Autodesk Inventor part; units mm, degrees
ref_plane "BODY_N_XY" through (62, 0, 0) normal (0, 0, -1) x (1, 0, 0)
ref_plane "BODY_N_YZ" through (62, 0, 0) normal (1, 0, 0) x (0, -1, 0)
ref_plane "BODY_N_ZX" through (62, 0, 0) normal (0, -1, 0) x (0, 0, -1)
sketch "Sketch_8" plane through (0, 0, 0) normal (0, 0, 1) x (1, 0, 0)
  line L0 (0, 0) -> (-8, 0)
  line L1 (-8, 0) -> (-8, 4.3865)
  line L2 (-8, 4.3865) -> (-7.3865, 5)
  line L3 (-7.3865, 5) -> (0, 5)
  line L4 (0, 5) -> (0, 0)
  line L5 (0, 0) -> (-8, 0)
revolve "Revolution1" add sketch "Sketch_8" angle 360 about axis through (0, 0, 0) along (1, 0, 0)
thread "Thread1"
sketch "Sketch_9" plane through (0, 0, 0) normal (1, 0, 0) x (0, 0, -1)
  line L0 (-9.15, 4.0345) -> (-9.15, -4.0345)
  arc A0 (-9.15, -4.0345) -> (-4.0345, -9.15) centre (0, 0) ccw
  line L1 (-4.0345, -9.15) -> (4.0345, -9.15)
  arc A1 (4.0345, -9.15) -> (9.15, -4.0345) centre (0, 0) ccw
  line L2 (9.15, -4.0345) -> (9.15, 4.0345)
  arc A2 (9.15, 4.0345) -> (4.0345, 9.15) centre (0, 0) ccw
  line L3 (4.0345, 9.15) -> (-4.0345, 9.15)
  arc A3 (-4.0345, 9.15) -> (-9.15, 4.0345) centre (0, 0) ccw
extrude "Extrusion1" add sketch "Sketch_9" along normal blind 12.5
sketch "Sketch_11" plane through (12.5, 0, 0) normal (1, 0, 0) x (0, 0, -1)
  circle A0 centre (0, 0) radius 8.7
extrude "Extrusion2" add sketch "Sketch_11" along normal blind 40
sketch "Sketch_10" plane through (52.5, 0, 0) normal (1, 0, 0) x (0, 0, -1)
  line L0 (-9.15, 4.0345) -> (-9.15, -4.0345)
  arc A0 (-9.15, -4.0345) -> (-4.0345, -9.15) centre (0, 0) ccw
  line L1 (-4.0345, -9.15) -> (4.0345, -9.15)
  arc A1 (4.0345, -9.15) -> (9.15, -4.0345) centre (0, 0) ccw
  line L2 (9.15, -4.0345) -> (9.15, 4.0345)
  arc A2 (9.15, 4.0345) -> (4.0345, 9.15) centre (0, 0) ccw
  line L3 (4.0345, 9.15) -> (-4.0345, 9.15)
  arc A3 (-4.0345, 9.15) -> (-9.15, 4.0345) centre (0, 0) ccw
extrude "Extrusion3" add sketch "Sketch_10" along normal blind 9.5
sketch "Sketch5" plane through (0, 9.15, 4.0345) normal (0, 1, 0) x (1, 0, 0)
  point P0 (8, 4.0345)
hole "Hole1" at (8, 9.15, 0) direction (0, -1, 0) diameter 4.134 depth 5 tip angle 120 countersink diameter 5 countersink angle 90
sketch "Sketch6" plane through (52.5, 9.15, 4.0345) normal (0, 1, 0) x (1, 0, 0)
  point P0 (4.5, 4.0345)
hole "Hole2" at (57, 9.15, 0) direction (0, -1, 0) diameter 4.134 depth 5 tip angle 120 countersink diameter 5 countersink angle 90
sketch "Sketch_16" plane through (0, 0, 0) normal (0, 0, 1) x (1, 0, 0)
  line L0 (32.5, 0) -> (-8, 0)
  line L1 (-8, 0) -> (-8, 2.5)
  line L2 (-8, 2.5) -> (12.5, 2.5)
  line L3 (12.5, 2.5) -> (12.5, 8)
  line L4 (12.5, 8) -> (32.5, 8)
  line L5 (32.5, 8) -> (32.5, 0)
  line L6 (32.5, 0) -> (-8, 0)
revolve "Revolution2" cut sketch "Sketch_16" angle 360 about axis through (32.5, 0, 0) along (1, 0, 0)
ref_plane "BODY_N_XY" through (62, 0, 0) normal (0, 0, -1) x (1, 0, 0)
ref_plane "BODY_N_YZ" through (62, 0, 0) normal (1, 0, 0) x (0, -1, 0)
ref_plane "BODY_N_ZX" through (62, 0, 0) normal (0, -1, 0) x (0, 0, -1)
ref_plane "NUT2_XY" through (62, 0, 0) normal (1, 0, 0) x (0, 0, -1)
ref_plane "NUT2_YZ" through (62, 0, 0) normal (0, 0, -1) x (0, 1, 0)
ref_plane "NUT2_ZX" through (62, 0, 0) normal (0, 1, 0) x (1, 0, 0)
ref_plane "SW1_XY" through (19, 0, 0) normal (1, 0, 0) x (0, 0, -1)
ref_plane "SW1_YZ" through (19, 0, 0) normal (0, 0, -1) x (0, 1, 0)
ref_plane "SW1_ZX" through (19, 0, 0) normal (0, 1, 0) x (1, 0, 0)
ref_plane "SW2_XY" through (46, 0, 0) normal (-1, 0, 0) x (0, 0, -1)
ref_plane "SW2_YZ" through (46, 0, 0) normal (0, 0, -1) x (0, -1, 0)
ref_plane "SW2_ZX" through (46, 0, 0) normal (0, -1, 0) x (-1, 0, 0)
ref_plane "SW_R1_XY" through (19, -14.15, 0) normal (1, 0, 0) x (0, 0, -1)
ref_plane "SW_R1_YZ" through (19, -14.15, 0) normal (0, 0, -1) x (0, 1, 0)
ref_plane "SW_R1_ZX" through (19, -14.15, 0) normal (0, 1, 0) x (1, 0, 0)
ref_plane "SW_R2_XY" through (46, -14.15, 0) normal (-1, 0, 0) x (0, 0, -1)
ref_plane "SW_R2_YZ" through (46, -14.15, 0) normal (0, 0, -1) x (0, -1, 0)
ref_plane "SW_R2_ZX" through (46, -14.15, 0) normal (0, -1, 0) x (-1, 0, 0)
ref_plane "body_XY" through (0, 0, 0) normal (-1, 0, 0) x (0, 0, -1)
ref_plane "body_YZ" through (0, 0, 0) normal (0, 0, -1) x (0, -1, 0)
ref_plane "body_ZX" through (0, 0, 0) normal (0, -1, 0) x (-1, 0, 0)
properties part number "CJ2B16-15Z-B(1_0)_BODY"
Source: CAD feature listing. Evaluate the final solid. Frame: model axes, mm. A direction names the side the tool comes from. Give positions to 0.01 mm unless a question says otherwise; leave off trailing zeros. Write each loop counter-clockwise with the first axis right and the second up, starting at its lowest first coordinate (ties: lowest second). Pieces come first, ordered by that corner, then holes. Notation, with made-up numbers: (18, 31.25) - (65, 31.25) arc R4 ccw to (65, 38.25) - close; hole circle Ø5 at (43, 35.25). An arc over 180 degrees is marked (long way). Write item = value, one per line. Start each with the question number.
Q1. Material intervals for probe 1 along X at (y, z) = (7.2, 0); probe 2 along X at (y, z) = (7.75, -5.5); probe 3 along X at (y, z) = (-0.25, 7.75), sorted ascending.
Q2. Cut plane B-B, the plane x = 15. Return loops of the section in (y, z).
Q3. Draft query along X for faces 1 (the flat face through (-8, 2, -2)), 2 (the cylindrical face through (6.16, 7.03, 7.11)), 3 (the cylindrical face through (9.26, 6.4, -1.64)). Return one class per face: +X half, -X half, draft (parallel to the pull), parting line (faces both ways), or undercut.
Q4. Cut plane A-A, the plane y = 0. Return loops of the section in (x, z), then the cut area to 3 significant figures.
Q5. Cut plane C-C, the plane x = 38. Return loops of the section in (y, z).
Q6. Reachability of faces 4 (the cylindrical face through (57.18, 7.03, 7.11)), 5 (the flat face through (52.5, -9, 1)), 6 (the cylindrical face through (54.95, 6.4, -0.27)), 7 (the cylindrical face through (-3.64, -1.08, -4.88)) from +Z, -Z, +X, -X, +Y, -Y: full face, straight path, thin tool, end or side. Return the list, or none.
Q7. Pin query (flat end, axial travel): pin 1 Ø2 at (y, z) = (-1.5, -5) entering from -X; pin 2 Ø1.5 at (x, z) = (48, 7) entering from +Y; pin 3 Ø5 at (x, z) = (36.5, -0.5) entering from +Y; pin 4 Ø2.5 at (x, z) = (8, 0) entering from +Y. Return the tip coordinate at first contact, or that it passes through.
Computed values:
q1.probe_1 = 0 to 5.93, 10.07 to 12.5, 32.5 to 54.93, 59.07 to 62
q1.probe_2 = 0 to 12.5, 52.5 to 62
q1.probe_3 = 0 to 12.5, 32.5 to 62
q2.outline = circle Ø17.4 at (0, 0); hole circle Ø16 at (0, 0)
q3.face_1 = -X half
q3.face_2 = draft
q3.face_3 = undercut
q4.outline = (-8, -4.39) - (-7.39, -5) - (0, -5) - (0, -9.15) - (12.5, -9.15) - (12.5, -8.7) - (52.5, -8.7) - (52.5, -9.15) - (62, -9.15) - (62, 9.15) - (52.5, 9.15) - (52.5, 8.7) - (12.5, 8.7) - (12.5, 9.15) - (0, 9.15) - (0, 5) - (-7.39, 5) - (-8, 4.39) - (-8, 2.5) - (12.5, 2.5) - (12.5, 8) - (32.5, 8) - (32.5, -8) - (12.5, -8) - (12.5, -2.5) - (-8, -2.5) - close
q4.area = 756 mm²
q5.outline = circle Ø17.4 at (0, 0)
q6.face_4 = +Z, +X, -X, +Y
q6.face_5 = none
q6.face_6 = +Y
q6.face_7 = -X
q7.pin_1 = -8
q7.pin_2 = 6.05
q7.pin_3 = 8.7
q7.pin_4 = 3.68
